Input: part model. Units: mm. Frame: model coordinates. A direction names the side the tool comes from. Coordinates: 2 decimals unless noted, no trailing zeros. Order: outer loops, then holes, each group sorted by start corner. A loop starts at its lowest first (then second) coordinate and runs counter-clockwise, first axis right, second up.
from build123d import *

# Parameters (mm, degrees)
SKETCH1_R           = 18
SKETCH1_R_2         = 3.5
SKETCH1_R_3         = 15
SKETCH1_R_4         = 8
SKETCH1_R_5         = 6
BOSS_EXTRUDE1_DEPTH = 5.5
SKETCH1_3_R         = 18
SKETCH1_3_R_2       = 15
BOSS_EXTRUDE2_DEPTH = 6
SKETCH1_4_R         = 15
SKETCH1_4_R_2       = 8
BOSS_EXTRUDE3_DEPTH = 5.5
SKETCH1_5_R         = 8
SKETCH1_5_R_2       = 6
BOSS_EXTRUDE4_DEPTH = 10.5
SKETCH2_R           = 15
SKETCH2_R_2         = 8
CUT_EXTRUDE1_DEPTH  = 0.5


with BuildPart() as part:
    # Sketch1 → Boss-Extrude1 (new body)
    # profile 1 of 4: a face of its own
    with BuildSketch(Plane(origin=(0, 0, 0), x_dir=(1, 0, 0), z_dir=(0, 1, 0))):
        with BuildLine():
            ThreePointArc((26.949557882, 6.895658656), (31.5, 0), (26.949557882, -6.895658656))
            Line((26.949557882, -6.895658656), (13.847382424, -12.5))
            ThreePointArc((13.847382424, -12.5), (0, -19), (-13.847382424, -12.5))
            Line((-13.847382424, -12.5), (-26.949557882, -6.895658656))
            ThreePointArc((-26.949557882, -6.895658656), (-31.5, 0), (-26.949557882, 6.895658656))
            Line((-26.949557882, 6.895658656), (-13.847382424, 12.5))
            ThreePointArc((-13.847382424, 12.5), (0, 19), (13.847382424, 12.5))
            Line((13.847382424, 12.5), (26.949557882, 6.895658656))
        make_face()
        Circle(SKETCH1_R, mode=Mode.SUBTRACT)
        with Locations(Location((-24, 0, 0), (0, 0, 270))):
            Circle(SKETCH1_R_2, mode=Mode.SUBTRACT)
        with Locations(Location((24, 0, 0), (0, 0, 270))):
            Circle(SKETCH1_R_2, mode=Mode.SUBTRACT)
    # profile 2 of 4: a face of its own
    with BuildSketch(Plane(origin=(0, 0, 0), x_dir=(1, 0, 0), z_dir=(0, 1, 0))):
        Circle(SKETCH1_R)
        Circle(SKETCH1_R_3, mode=Mode.SUBTRACT)
    # profile 3 of 4: a face of its own
    with BuildSketch(Plane(origin=(0, 0, 0), x_dir=(1, 0, 0), z_dir=(0, 1, 0))):
        Circle(SKETCH1_R_3)
        Circle(SKETCH1_R_4, mode=Mode.SUBTRACT)
    # profile 4 of 4: a face of its own
    with BuildSketch(Plane(origin=(0, 0, 0), x_dir=(1, 0, 0), z_dir=(0, 1, 0))):
        Circle(SKETCH1_R_4)
        with Locations(Location((0, 0, 0), (0, 0, 270))):
            Circle(SKETCH1_R_5, mode=Mode.SUBTRACT)
    extrude(amount=-BOSS_EXTRUDE1_DEPTH)

    # Sketch1_3 → Boss-Extrude2 (add)
    with BuildSketch(Plane(origin=(0, 0, 0), x_dir=(1, 0, 0), z_dir=(0, 1, 0))):
        with Locations(Location((0, 0, 0), (0, 0, 270))):
            Circle(SKETCH1_3_R)
        with Locations(Location((0, 0, 0), (0, 0, 270))):
            Circle(SKETCH1_3_R_2, mode=Mode.SUBTRACT)
    extrude(amount=BOSS_EXTRUDE2_DEPTH)

    # Sketch1_4 → Boss-Extrude3 (add)
    with BuildSketch(Plane(origin=(0, 0, 0), x_dir=(1, 0, 0), z_dir=(0, 1, 0))):
        with Locations(Location((0, 0, 0), (0, 0, 270))):
            Circle(SKETCH1_4_R)
        with Locations(Location((0, 0, 0), (0, 0, 270))):
            Circle(SKETCH1_4_R_2, mode=Mode.SUBTRACT)
    extrude(amount=BOSS_EXTRUDE3_DEPTH)

    # Sketch1_5 → Boss-Extrude4 (add)
    with BuildSketch(Plane(origin=(0, 0, 0), x_dir=(1, 0, 0), z_dir=(0, 1, 0))):
        with Locations(Location((0, 0, 0), (0, 0, 90))):
            Circle(SKETCH1_5_R)
        with Locations(Location((0, 0, 0), (0, 0, 270))):
            Circle(SKETCH1_5_R_2, mode=Mode.SUBTRACT)
    extrude(amount=BOSS_EXTRUDE4_DEPTH)

    # Sketch2 → Cut-Extrude1 (cut)
    with BuildSketch(Plane.XZ.offset(5.5)):
        with Locations(Location((0, 0, 0), (0, 0, 90))):
            Circle(SKETCH2_R)
        with Locations(Location((0, 0, 0), (0, 0, 270))):
            Circle(SKETCH2_R_2, mode=Mode.SUBTRACT)
    extrude(amount=-CUT_EXTRUDE1_DEPTH, mode=Mode.SUBTRACT)


solid = part.part
Item 1: Access query for faces 5 (the face through (-7.81, -5.25, 1.73)), 6 (the face through (7.81, 7.96, 1.73)), 7 (the face through (-2, -5.5, -6)). Directions: +Z, -Z, +X, -X, +Y, -Y. A direction counts if a zero-diameter tool reaches every point of the face in a straight line with its end or side. Return the directions, or none.
Response values:
face 5: -Y
face 6: +Y
face 7: +Z, -Z, +X, -X, -Y
Item 2: Cut plane C-C on z = 0. Count the separate pieces of the cut face and the enclosed holes in it, then the cut area to 4 significant figures.
Response values:
separate pieces: 4
enclosed holes: 0
area: 351.5 mm2
Item 3: Cut plane A-A on y = -2. Return loops of the section in (x, z).
Response values:
outline: (-26.95, -6.9) - (-13.85, -12.5) arc R18 ccw to (13.85, -12.5) - (26.95, -6.9) arc R7.5 ccw to (26.95, 6.9) - (13.85, 12.5) arc R18 ccw to (-13.85, 12.5) - (-26.95, 6.9) arc R7.5 ccw to start; hole circle Ø7 at (-24, 0); hole circle Ø12 at (0, 0); hole circle Ø7 at (24, 0)
Item 4: Cut plane B-B on x = -24. Return loops of the section in (y, z), then the cut area to 3 significant figures.
Response values:
outline: (-5.5, -8.16) - (0, -8.16) - (0, -3.5) - (-5.5, -3.5) - close; (-5.5, 3.5) - (0, 3.5) - (0, 8.16) - (-5.5, 8.16) - close
area: 51.2 mm2
Item 5: Draft query along X for faces 1 (the face through (6, -5, 6)), 2 (the face through (-20.49, -2.71, -9.66)), 3 (the face through (-20.53, -2.71, -0.46)), 4 (the face through (5.407, 2.958, 17.169)). Return one class per face: pulls with the +X half, pulls with the -X half, needs draft (parallel to the pull), parting line crosses it, or undercut.
Response values:
face 1: undercut
face 2: pulls with the -X half
face 3: undercut
face 4: parting line crosses it
Item 6: Pin query (flat end, axial travel): pin 1 Ø4 at (x, y) = (6.5, 7.5) entering from +Z; pin 2 Ø11 at (x, z) = (-24, 0) entering from +Y; pin 3 Ø3 at (y, z) = (0, 9.5) entering from +X. Return the tip coordinate at first contact, or that it passes through.
Response values:
pin 1: stops at z = 17.24
pin 2: stops at y = 0
pin 3: stops at x = 24.37
Item 7: Cut plane D-D on y = 9.75. Return loops of the section in (x, z), then the cut area to 3 significant figures.
Response values:
outline: circle Ø16 at (0, 0); hole circle Ø12 at (0, 0)
area: 88.0 mm2
Item 8: Ray query, probe 1 along X at (y, z) = (5, 0); probe 2 along Y at (x, z) = (-3, -14.5); probe 3 along X at (y, z) = (8.75, -4.5). Return the intervals inside material, ascending.
Response values:
probe 1: x = -18 to -6, 6 to 18
probe 2: y = -5 to 5.5
probe 3: x = -6.61 to -3.97, 3.97 to 6.61
